```python
from build123d import *

# Parameters (mm, degrees)
SKETCH1_R           = 12.7
SKETCH1_R_2         = 10.287
BOSS_EXTRUDE1_DEPTH = 24.384
SKETCH2_R           = 14.4526
SKETCH2_R_2         = 10.287
BOSS_EXTRUDE2_DEPTH = 1.524
CHAMFER1_SIZE       = 0.508


with BuildPart() as part:
    # Sketch1 → Boss-Extrude1 (new body)
    with BuildSketch(Plane(origin=(0, 0, 0), x_dir=(1, 0, 0), z_dir=(0, 1, 0))):
        with Locations(Location((0, 0, 0), (0, 0, 90))):
            Circle(SKETCH1_R)
        with Locations(Location((0, 0, 0), (0, 0, 90))):
            Circle(SKETCH1_R_2, mode=Mode.SUBTRACT)
    extrude(amount=BOSS_EXTRUDE1_DEPTH)

    # Sketch2 → Boss-Extrude2 (add)
    with BuildSketch(Plane(origin=(0, 24.384, 0), x_dir=(1, 0, 0), z_dir=(0, 1, 0))):
        with Locations(Location((0, 0, 0), (0, 0, 90))):
            Circle(SKETCH2_R)
        with Locations(Location((0, 0, 0), (0, 0, 90))):
            Circle(SKETCH2_R_2, mode=Mode.SUBTRACT)
    extrude(amount=BOSS_EXTRUDE2_DEPTH)

    # Chamfer1
    chamfer1_edges = [part.edges().sort_by_distance(p)[0] for p in [
        (0, 25.908, 10.287),
        (0, 0, 10.287),
    ]]
    chamfer(chamfer1_edges, length=CHAMFER1_SIZE)


solid = part.part
```
Work out the finished part from the listing and answer in its coordinate system (mm). Coordinates: 2 decimals unless noted, no trailing zeros. Write each loop counter-clockwise with the first axis right and the second up, starting at its lowest first coordinate (ties: lowest second). Pieces come first, ordered by that corner, then holes.
Q1. Determine the mould class of faces 1 (the face through (13, 24.384, 0)), 2 (the face through (-10.2, 12.78, 1.34)), 3 (the face through (7.7, 12, 10.1)) for opening direction Z: released by +Z, released by -Z, zero draft, split by the parting line, or undercut.
Q2. Each of these flat-tipped pins is pushed along its axis until it touches: pin 1 Ø1 at (x, y) = (-5.5, 21) entering from +Z; pin 2 Ø8 at (x, y) = (-4, 13) entering from +Z; pin 3 Ø5 at (x, z) = (-7, 6.5) entering from +Y; pin 4 Ø4 at (x, z) = (7, 2) entering from -Y. Where does it stop, or does it pass through?
Q3. A cutting plane is placed at A-A, the plane z = 0. Give the vertices of the cut face in (x, y) (3 decimals).
Q4. A cutting plane is placed at C-C, the plane y = 3. Give the vertices of the cut face in (x, z).
Q5. A cutting plane is placed at B-B, the plane x = 0. Give the vertices of the cut face in (y, z) (3 decimals).
Q6. A cutting plane is placed at D-D, the plane z = -11.75. Give the vertices of the cut face in (x, y), then the cut area to 3 significant figures.
Q7. Find the intervals of material crossed by line 1 (X direction, y = 15, z = 0); line 2 (Z direction, x = 0.25, y = 11.5); line 3 (Y direction, x = 9.25, z = 10.75), in increasing order.
Findings below:
1. face 1: zero draft
1. face 2: undercut
1. face 3: split by the parting line
2. pin 1: stops at z = 11.67
2. pin 2: stops at z = 12.7
2. pin 3: stops at y = 25.91
2. pin 4: passes through
3. outline: (-14.453, 24.384) - (-12.7, 24.384) - (-12.7, 0) - (-10.795, 0) - (-10.287, 0.508) - (-10.287, 25.4) - (-10.795, 25.908) - (-14.453, 25.908) - close; (10.287, 0.508) - (10.795, 0) - (12.7, 0) - (12.7, 24.384) - (14.453, 24.384) - (14.453, 25.908) - (10.795, 25.908) - (10.287, 25.4) - close
4. outline: circle Ø25.4 at (0, 0); hole circle Ø20.57 at (0, 0)
5. outline: (0, -12.7) - (24.384, -12.7) - (24.384, -14.453) - (25.908, -14.453) - (25.908, -10.795) - (25.4, -10.287) - (0.508, -10.287) - (0, -10.795) - close; (0, 10.795) - (0.508, 10.287) - (25.4, 10.287) - (25.908, 10.795) - (25.908, 14.453) - (24.384, 14.453) - (24.384, 12.7) - (0, 12.7) - close
6. outline: (-8.42, 24.38) - (-4.82, 24.38) - (-4.82, 0) - (4.82, 0) - (4.82, 24.38) - (8.42, 24.38) - (8.42, 25.91) - (-8.42, 25.91) - close
6. area: 261 mm2
7. line 1: x = -12.7 to -10.29, 10.29 to 12.7
7. line 2: z = -12.7 to -10.28, 10.28 to 12.7
7. line 3: y = 24.38 to 25.91
